Check sheet for the modelled part. Datum: model origin and axes. Units: mm. Round coordinates to 2 decimals unless told otherwise and drop trailing zeros. Write each loop counter-clockwise with the first axis right and the second up, starting at its lowest first coordinate (ties: lowest second). Pieces come first, ordered by that corner, then holes.
Item 1: Material ranges on line 1 along Y through (x, z) = (-38, 1.25); line 2 along Y through (x, z) = (13.5, 0.55); line 3 along X through (y, z) = (-136, 1.7), recorded low to high.
Item 2: Section check C-C, the plane y = -136. Record the cut outline in (x, z).
Item 3: Section check A-A, the plane y = 127. Record the cut outline in (x, z).
Item 4: Depth check by flat-ended pin: pin 1 (0.6 mm diameter, centred on x = 39, z = 0.5, fed in from +Y); pin 2 (1 mm diameter, centred on x = 4.5, z = 1.5, fed in from +Y). Enter the tip coordinate at first touch or a pass-through.
Item 5: Section check B-B, the plane x = -5.5. Record the cut outline in (y, z), plus the area to 3 significant figures.
from build123d import *

# Parameters (mm, degrees)
BOSS_EXTRUDE1_DEPTH = 2
FILLET1_R           = 3


with BuildPart() as part:
    # Sketch2 → Boss-Extrude1 (new body)
    with BuildSketch(Plane.XY):
        with BuildLine():
            Line((-25, -165.5), (25, -165.5))
            ThreePointArc((25, -165.5), (31.01040764, -167.98959236), (33.5, -174))
            Line((33.5, -174), (66.5, -174))
            ThreePointArc((66.5, -174), (75, -165.5), (83.5, -174))
            Line((83.5, -174), (174, -174))
            Line((174, -174), (174, -143))
            ThreePointArc((174, -143), (165.5, -134.5), (174, -126))
            Line((174, -126), (174, 174))
            Line((174, 174), (83.5, 174))
            ThreePointArc((83.5, 174), (75, 165.5), (66.5, 174))
            Line((66.5, 174), (45, 174))
            Line((45, 174), (45, 165.5))
            Line((45, 165.5), (27.5, 165.5))
            Line((27.5, 165.5), (27.5, 104))
            Line((27.5, 104), (-27.5, 104))
            Line((-27.5, 104), (-27.5, 165.5))
            Line((-27.5, 165.5), (-45, 165.5))
            Line((-45, 165.5), (-45, 174))
            Line((-45, 174), (-66.5, 174))
            ThreePointArc((-66.5, 174), (-75, 165.5), (-83.5, 174))
            Line((-83.5, 174), (-174, 174))
            Line((-174, 174), (-174, -126))
            ThreePointArc((-174, -126), (-165.5, -134.5), (-174, -143))
            Line((-174, -143), (-174, -174))
            Line((-174, -174), (-83.5, -174))
            ThreePointArc((-83.5, -174), (-75, -165.5), (-66.5, -174))
            Line((-66.5, -174), (-33.5, -174))
            ThreePointArc((-33.5, -174), (-31.01040764, -167.98959236), (-25, -165.5))
        make_face()
    extrude(amount=BOSS_EXTRUDE1_DEPTH)

    # Fillet1
    fillet1_edges = [part.edges().sort_by_distance(p)[0] for p in [
        (174, -174, 1),
        (83.5, -174, 1),
        (66.5, -174, 1),
        (33.5, -174, 1),
        (-33.5, -174, 1),
        (-66.5, -174, 1),
        (-83.5, -174, 1),
        (-174, -174, 1),
        (-174, -143, 1),
        (-174, -126, 1),
        (-174, 174, 1),
        (-83.5, 174, 1),
        (-66.5, 174, 1),
        (-45, 174, 1),
        (-45, 165.5, 1),
        (-27.5, 165.5, 1),
        (-27.5, 104, 1),
        (27.5, 104, 1),
        (27.5, 165.5, 1),
        (45, 165.5, 1),
        (45, 174, 1),
        (66.5, 174, 1),
        (83.5, 174, 1),
        (174, 174, 1),
        (174, -126, 1),
        (174, -143, 1),
    ]]
    fillet(fillet1_edges, radius=FILLET1_R)


solid = part.part
Values found:
1. line 1: y = -174 to 165.5
1. line 2: y = -165.5 to 104
1. line 3: x = -165.63 to 165.63
2. outline: (-165.63, 0) - (165.63, 0) - (165.63, 2) - (-165.63, 2) - close
3. outline: (-174, 0) - (-27.5, 0) - (-27.5, 2) - (-174, 2) - close; (27.5, 0) - (174, 0) - (174, 2) - (27.5, 2) - close
4. pin 1: stops at y = 165.5
4. pin 2: stops at y = 104
5. outline: (-165.5, 0) - (104, 0) - (104, 2) - (-165.5, 2) - close
5. area: 539 mm2
